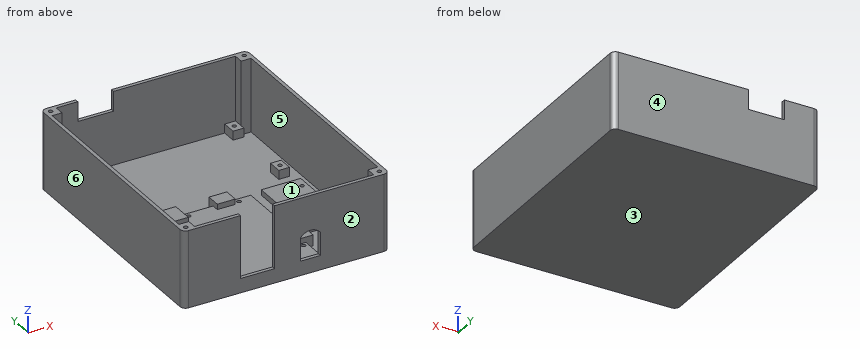
from build123d import *

# Parameters (mm, degrees)
F0_W      = 115
F0_H      = 137
F1_DEPTH  = 2
F2_W      = 115
F2_H      = 137
F2_W_2    = 111
F2_H_2    = 133
F3_DEPTH  = 41
F4_W      = 6
F4_H      = 8
F4_R      = 1.15
F5_DEPTH  = 5
F6_W      = 22
F6_H      = 43
F6_R      = 1.15
F7_DEPTH  = 3
F8_W      = 53.5
F8_H      = 69
F8_R      = 1.15
F9_DEPTH  = 3
F10_W     = 10
F10_H     = 8
F10_W_2   = 7
F10_H_2   = 10
F10_H_3   = 12
F11_DEPTH = 6
F12_W     = 19
F12_H     = 5.221757
F12_H_2   = 32
F13_DEPTH = 2
F14_W     = 20
F14_H     = 11
F15_DEPTH = 2
F16_W     = 5.5
F16_H     = 5.5
F17_DEPTH = 41
F18_R     = 1.15
F19_DEPTH = 5
F20_R     = 3


with BuildPart() as f1:
    # F0 (on Top) → F1 (new body)
    with BuildSketch(Plane.XY):
        Rectangle(F0_W, F0_H)
    extrude(amount=F1_DEPTH)

    # F2 (on face) → F3 (join)
    with BuildSketch(Plane.XY.offset(2)):
        Rectangle(F2_W, F2_H)
        Rectangle(F2_W_2, F2_H_2, mode=Mode.SUBTRACT)
    extrude(amount=F3_DEPTH)

    # F4 (on face) → F5 (join)
    with BuildSketch(Plane.XY.offset(2)):
        with Locations((-47, 62.5)):
            Rectangle(F4_W, F4_H)
        with Locations((-47, 62.5)):
            Circle(F4_R, mode=Mode.SUBTRACT)
        with Locations((47, 62.5)):
            Rectangle(F4_W, F4_H)
        with Locations((47, 62.5)):
            Circle(F4_R, mode=Mode.SUBTRACT)
        with Locations((-47, 18.5)):
            Rectangle(F4_W, F4_H)
        with Locations((-47, 18.5)):
            Circle(F4_R, mode=Mode.SUBTRACT)
        with Locations((47, 18.5)):
            Rectangle(F4_W, F4_H)
        with Locations((47, 18.5)):
            Circle(F4_R, mode=Mode.SUBTRACT)
    extrude(amount=F5_DEPTH)

    # F6 (on face) → F7 (join)
    with BuildSketch(Plane.XY.offset(2)):
        with Locations((40, -16)):
            Rectangle(F6_W, F6_H)
        with Locations((32, -31)):
            Circle(F6_R, mode=Mode.SUBTRACT)
        with Locations((48, -1)):
            Circle(F6_R, mode=Mode.SUBTRACT)
    extrude(amount=F7_DEPTH)

    # F8 (on face) → F9 (join)
    with BuildSketch(Plane.XY.offset(2)):
        with Locations((-4.75, -31)):
            Rectangle(F8_W, F8_H)
        with Locations((19.5, -51.5)):
            Circle(F8_R, mode=Mode.SUBTRACT)
        with Locations((-14, 1)):
            Circle(F8_R, mode=Mode.SUBTRACT)
        with Locations((14, 1)):
            Circle(F8_R, mode=Mode.SUBTRACT)
    extrude(amount=F9_DEPTH)

    # F10 (on face) → F11 (join)
    with BuildSketch(Plane.XY.offset(2)):
        with Locations((6, 3.5)):
            Rectangle(F10_W, F10_H)
        with Locations((21, -45.5)):
            Rectangle(F10_W, F10_H)
        with Locations((-28, -60.5)):
            Rectangle(F10_W_2, F10_H_2)
        with Locations((-22.5, 1.5)):
            Rectangle(F10_W, F10_H_3)
    extrude(amount=F11_DEPTH)

    # F12 (on face) → F13 (cut)
    with BuildSketch(Plane(origin=(0, -66.5, 0), x_dir=(-1, 0, 0), z_dir=(0, 1, 0))):
        with Locations((16, 42.610878)):
            Rectangle(F12_W, F12_H)
        with Locations((16, 24)):
            Rectangle(F12_W, F12_H_2)
        with BuildLine():
            Line((-19, 8), (-8, 8))
            Line((-8, 8), (-8, 21))
            ThreePointArc((-8, 21), (-13.5, 23.669873), (-19, 21))
            Line((-19, 21), (-19, 8))
        make_face()
    extrude(amount=-F13_DEPTH, mode=Mode.SUBTRACT)

    # F14 (on face) → F15 (cut)
    with BuildSketch(Plane(origin=(0, 68.5, 0), x_dir=(-1, 0, 0), z_dir=(0, 1, 0))):
        with Locations((28, 37.5)):
            Rectangle(F14_W, F14_H)
    extrude(amount=-F15_DEPTH, mode=Mode.SUBTRACT)

    # F16 (on face) → F17 (join)
    with BuildSketch(Plane.XY.offset(2)):
        with Locations((-52.75, -63.75)):
            Rectangle(F16_W, F16_H)
        with Locations((-52.75, 63.75)):
            Rectangle(F16_W, F16_H)
        with Locations((52.75, 63.75)):
            Rectangle(F16_W, F16_H)
        with Locations((52.75, -63.75)):
            Rectangle(F16_W, F16_H)
    extrude(amount=F17_DEPTH)

    # F18 (on face) → F19 (cut)
    with BuildSketch(Plane.XY.offset(43)):
        with Locations((-54, -65)):
            Circle(F18_R)
        with Locations((-54, 65)):
            Circle(F18_R)
        with Locations((54, 65)):
            Circle(F18_R)
        with Locations((54, -65)):
            Circle(F18_R)
    extrude(amount=-F19_DEPTH, mode=Mode.SUBTRACT)

    # F20
    f20_edges = [f1.edges().sort_by_distance(p)[0] for p in [
        (-57.5, -68.5, 21.5),
        (57.5, -68.5, 21.5),
        (57.5, 68.5, 21.5),
        (-57.5, 68.5, 21.5),
    ]]
    fillet(f20_edges, radius=F20_R)


solid = f1.part
For this review, take the finished solid that the model builds, in its own axes (mm). Face numbers are marked on the shaded views. A direction names the side the tool comes from. Coordinates: 2 decimals unless noted, no trailing zeros. Order: outer loops, then holes, each group sorted by start corner. A loop starts at its lowest first (then second) coordinate and runs counter-clockwise, first axis right, second up. Notation, with made-up numbers: (62.5, 83) - (72.5, 83) arc R29 cw to (72.5, 111) - close; hole circle Ø2 at (72.5, 81.5). An arc over 180 degrees is marked (long way). Answer as CSV lines item,"result". Start each with the question number.
1) To check wall thickness, follow line 1 along Y through (x, z) = (-54, 40.25); line 2 along Y through (x, z) = (-28, 2.5); line 3 along Y through (x, z) = (32, 3). State the ranges of each line that lie inside material, in increasing order. Write a range as [from, to].
2) Machinability: for the marked faces 5 and 6, which of the approach directions +Z, -Z, +X, -X, +Y, -Y give a long, thin tool a straight path to every point of the face, cutting with its end or side? Answer none if there is none.
3) Add section D-D (x = 42). State the section outline as (y, z) points, then the cut area to 3 significant figures.
4) Insertion check: P1, Ø2.5, axis at x = 47, y = 18.5, coming from the +Z side; P2, Ø2.5, axis at x = 54, y = 65, coming from the +Z side; P3, Ø1.1, axis at x = -46.5, y = 62.5, coming from the +Z side; P4, Ø1.6, axis at x = -16, y = -68, coming from the +Z side. Each pin has a flat end and moves straight along its axis. Give the tip position at first contact, or say it passes through.
5) Add section B-B (z = 16). State the section outline as (x, y) points.
6) Add section A-A (z = 40). Count the separate pieces of the cut face and the enclosed holes in it, then the cut area to 3 significant figures.
7) Draft analysis for pull direction Y (two halves, no side actions). For the marked faces 1, 2, 3 and 4, state which applies: +Y half, -Y half, draft (parallel to the pull), parting line (faces both ways), or undercut.
8) Add section C-C (y = -22). State the section outline as (x, z) points, then the cut area to 4 significant figures.
Result:
1,line 1,"[-68.5, -66.15], [-63.85, -61], [61, 63.85], [66.15, 68.5]"
1,line 2,"[-68.5, -66.5], [-65.5, 3.5], [66.5, 68.5]"
1,line 3,"[-68.5, -66.5], [-37.5, -32.15], [-29.85, 5.5], [66.5, 68.5]"
2,face 5,"+Z"
2,face 6,"+Z, -Z, -X, +Y, -Y"
3,outline,"(-68.5, 0) - (68.5, 0) - (68.5, 43) - (66.5, 43) - (66.5, 2) - (5.5, 2) - (5.5, 5) - (-37.5, 5) - (-37.5, 2) - (-66.5, 2) - (-66.5, 43) - (-68.5, 43) - close"
3,area,"567 mm^2"
4,P1,"z = 7"
4,P2,"z = 43"
4,P3,"z = 2"
4,P4,"z = 8"
5,outline,"(-57.5, -65.5) arc R3 ccw to (-54.5, -68.5) - (-25.5, -68.5) - (-25.5, -66.5) - (-50, -66.5) - (-50, -61) - (-55.5, -61) - (-55.5, 61) - (-50, 61) - (-50, 66.5) - (50, 66.5) - (50, 61) - (55.5, 61) - (55.5, -61) - (50, -61) - (50, -66.5) - (19, -66.5) - (19, -68.5) - (54.5, -68.5) arc R3 ccw to (57.5, -65.5) - (57.5, 65.5) arc R3 ccw to (54.5, 68.5) - (-54.5, 68.5) arc R3 ccw to (-57.5, 65.5) - close; (-6.5, -68.5) - (8, -68.5) - (8, -66.5) - (-6.5, -66.5) - close"
6,separate pieces,"2"
6,enclosed holes,"4"
6,area,"1,010 mm^2"
7,face 1,"undercut"
7,face 2,"-Y half"
7,face 3,"draft"
7,face 4,"+Y half"
8,outline,"(-57.5, 0) - (57.5, 0) - (57.5, 43) - (55.5, 43) - (55.5, 2) - (51, 2) - (51, 5) - (29, 5) - (29, 2) - (22, 2) - (22, 5) - (-31.5, 5) - (-31.5, 2) - (-55.5, 2) - (-55.5, 43) - (-57.5, 43) - close"
8,area,"620.5 mm^2"
